Can you work these out from the drawing? Everything is in mm from the part's minimum corner. A direction names the side the tool comes from. Round coordinates to 2 decimals unless told otherwise and drop trailing zeros. Answer as a JSON object with one key per item and string values.
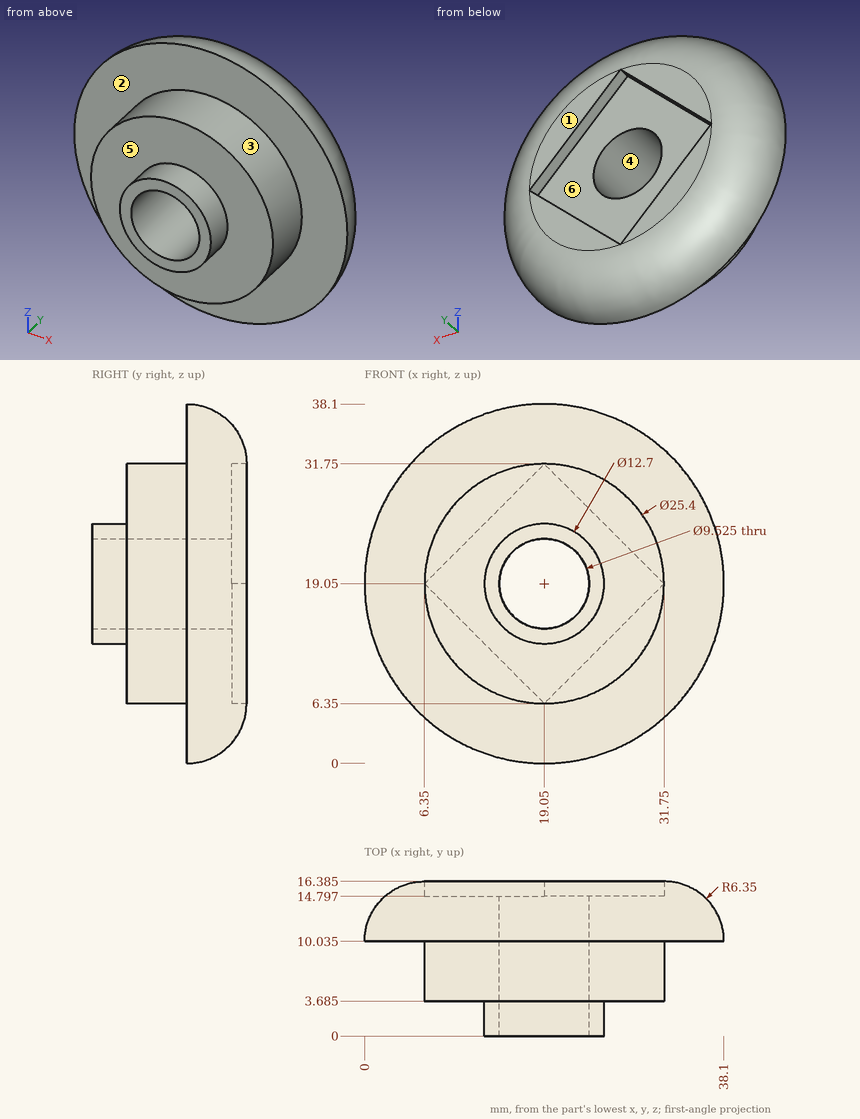
Q1. On a 3-axis mill with a long thin cutter (end or side, diameter ignored), from which of +Z, -Z, +X, -X, +Y, -Y can I reach the whole of each face in a straight line? I mean the marked faces 1 and 2. Say none if no direction works.
Determined:
{"face 1": "+Z, -Z, +X, -X, +Y", "face 2": "-Y"}
Q2. If I drill on L1, parallel to Z at x = 19.05, y = 5.5; L2, parallel to Y at x = 20, z = 26.5 (1 decimal); L3, parallel to Y at x = 26.5, z = 28.5 (1 decimal), over which ranges is the centre line in solid material (lowest first)? Write a range as [from, to].
Determined:
{"L1": "[6.35, 14.29], [23.81, 31.75]", "L2": "[3.7, 14.8]", "L3": "[3.7, 16.4]"}
Q3. We'd pull the mould along X, two halves only. Please class the marked faces 3, 4, 5 and 6: pulls with the +X half, pulls with the -X half, needs draft (parallel to the pull), parting line crosses it, or undercut.
Determined:
{"face 3": "parting line crosses it", "face 4": "undercut", "face 5": "needs draft", "face 6": "undercut"}
Q4. I'm going to push flat-ended pins straight in: pin 1 (3 mm diameter, centred on x = 16.5, y = 9, fed in from -Z); pin 2 (12.5 mm diameter, centred on x = 19.05, z = 19.05, fed in from +Y); pin 3 (8 mm diameter, centred on y = 13, z = 25.5, fed in from -X). Where does each tip first touch, or does it pass through?
Determined:
{"pin 1": "z = 0.06", "pin 2": "y = 14.8", "pin 3": "x = 0.3"}
